Part model, mm, in its own coordinate system. Face numbers are marked on the shaded views. A direction names the side the tool comes from. Give positions to 0.01 mm unless a question says otherwise; leave off trailing zeros. Order: outer loops, then holes, each group sorted by start corner. A loop starts at its lowest first (then second) coordinate and runs counter-clockwise, first axis right, second up. Notation, with made-up numbers: (-8, 63) - (35, 63) arc R16 cw to (35, 90) - close; hole circle Ø11 at (45.5, 45). An arc over 180 degrees is marked (long way). One line per item, written item: value.
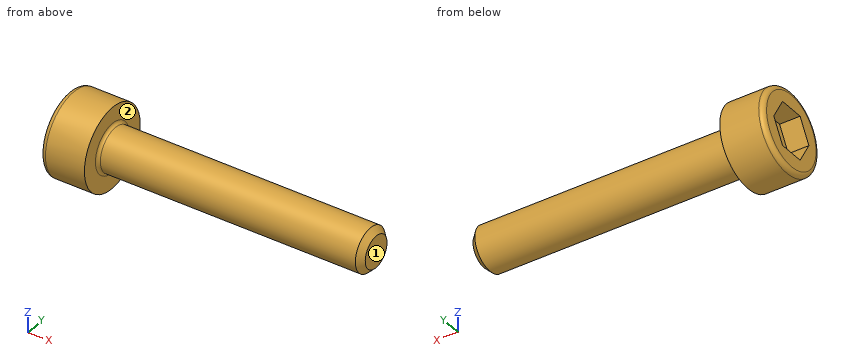
```python
from build123d import *

# Parameters (mm, degrees)
FILLET1_R      = 0.1
FILLET2_R      = 0.16
CHAMFER1_SIZE  = 0.2
EXTRUDE1_DEPTH = 0.7


with BuildPart() as part:
    # Sketch1 → Revolve1 (revolve)
    with BuildSketch(Plane.XY, mode=Mode.PRIVATE) as revolve1_sk:
        Polygon((0, 1.395688245), (0, 0), (10.488734128, 0), (10.488734128, 0.744367064), (1.488734128, 0.744367064), (1.488734128, 1.395688245), align=None)
    revolve(revolve1_sk.sketch.rotate(Axis((0, 0, 0), (1, 0, 0)), 90), axis=Axis((0, 0, 0), (1, 0, 0)))

    # Fillet1
    fillet1_edges = [part.edges().sort_by_distance(p)[0] for p in [
        (1.488734128, 0, -0.744367064),
    ]]
    fillet(fillet1_edges, radius=FILLET1_R)

    # Fillet2
    fillet2_edges = [part.edges().sort_by_distance(p)[0] for p in [
        (0, 0, -1.395688245),
    ]]
    fillet(fillet2_edges, radius=FILLET2_R)

    # Chamfer1
    chamfer1_edges = [part.edges().sort_by_distance(p)[0] for p in [
        (10.488734128, 0, -0.744367064),
    ]]
    chamfer(chamfer1_edges, length=CHAMFER1_SIZE)

    # Sketch2 → Extrude1 (cut)
    with BuildSketch(Plane.ZY):
        Polygon((0, 0.877572409), (-0.76, 0.438786205), (-0.76, -0.438786205), (0, -0.877572409), (0.76, -0.438786205), (0.76, 0.438786205), align=None)
    extrude(amount=-EXTRUDE1_DEPTH, mode=Mode.SUBTRACT)


solid = part.part
```
1) Cut at B-B, the plane x = 8. Give the cut face in (y, z), then the cut area to 3 significant figures.
Outcome:
outline: circle Ø1.49 at (0, 0)
area: 1.74 mm^2
2) Cut at A-A, the plane y = 0. Give the cut face in (x, z), then the cut area to 3 significant figures.
Outcome:
outline: (0, -1.24) arc R0.16 ccw to (0.16, -1.4) - (1.49, -1.4) - (1.49, -0.84) arc R0.1 cw to (1.59, -0.74) - (10.29, -0.74) - (10.49, -0.54) - (10.49, 0.54) - (10.29, 0.74) - (1.59, 0.74) arc R0.1 cw to (1.49, 0.84) - (1.49, 1.4) - (0.16, 1.4) arc R0.16 ccw to (0, 1.24) - (0, 0.76) - (0.7, 0.76) - (0.7, -0.76) - (0, -0.76) - close
area: 16.4 mm^2
3) Drill centre lines: line 1 along X through (y, z) = (0.15, 1.15); line 2 along X through (y, z) = (0.15, -0.4); line 3 along Z through (x, y) = (1.75, 0.6). Where is each one in solid material? Low to high. Write a range as from..to.
Outcome:
line 1: x = 0..1.49
line 2: x = 0.7..10.49
line 3: z = -0.44..0.44
4) Which spindle directions (+Z, -Z, +X, -X, +Y, -Y) get a long thin tool onto all of the face, cutting with end or side? Do the marked faces 1 and 2. Say none if no direction does.
Outcome:
face 1: +Z, -Z, +X, +Y, -Y
face 2: +X
